from build123d import *

# Parameters (mm, degrees)
BOSS_EXTRUDE2_DEPTH = 10
SKETCH3_R           = 3.5
BOSS_EXTRUDE3_DEPTH = 60
SKETCH4_R           = 3.5
BOSS_EXTRUDE4_DEPTH = 10


with BuildPart() as part:
    # Sketch1 → Boss-Extrude2 (new body)
    with BuildSketch(Plane.XY):
        with BuildLine():
            Line((0, 22.75), (0, -22.75))
            ThreePointArc((0, -22.75), (-0.292893219, -23.457106781), (-1, -23.75))
            Line((-1, -23.75), (-29, -23.75))
            ThreePointArc((-29, -23.75), (-29.707106781, -23.457106781), (-30, -22.75))
            Line((-30, -22.75), (-30, -14.75))
            ThreePointArc((-30, -14.75), (-29.707106781, -14.042893219), (-29, -13.75))
            Line((-29, -13.75), (-11, -13.75))
            ThreePointArc((-11, -13.75), (-10.292893219, -13.457106781), (-10, -12.75))
            Line((-10, -12.75), (-10, 32.75))
            ThreePointArc((-10, 32.75), (-9.707106781, 33.457106781), (-9, 33.75))
            Line((-9, 33.75), (19, 33.75))
            ThreePointArc((19, 33.75), (19.707106781, 33.457106781), (20, 32.75))
            Line((20, 32.75), (20, 24.75))
            ThreePointArc((20, 24.75), (19.707106781, 24.042893219), (19, 23.75))
            Line((19, 23.75), (1, 23.75))
            ThreePointArc((1, 23.75), (0.292893219, 23.457106781), (0, 22.75))
        make_face()
    extrude(amount=BOSS_EXTRUDE2_DEPTH)

    # Sketch3 → Boss-Extrude3 (add)
    with BuildSketch(Plane(origin=(20, 0, 0), x_dir=(0, 0, -1), z_dir=(1, 0, 0))):
        with Locations(Location((-5, 28.75, 0), (0, 0, 270))):
            Circle(SKETCH3_R)
    extrude(amount=BOSS_EXTRUDE3_DEPTH)

    # Sketch4 → Boss-Extrude4 (add)
    with BuildSketch(Plane.ZY.offset(30)):
        with Locations(Location((5, -18.75, 0), (0, 0, 90))):
            Circle(SKETCH4_R)
    extrude(amount=BOSS_EXTRUDE4_DEPTH)


solid = part.part
Work out the finished part from the listing and answer in its coordinate system (mm). A direction names the side the tool comes from. Round coordinates to 2 decimals unless told otherwise and drop trailing zeros. Write each loop counter-clockwise with the first axis right and the second up, starting at its lowest first coordinate (ties: lowest second). Pieces come first, ordered by that corner, then holes. Notation, with made-up numbers: (75, 19.5) - (80, 19.5) arc R15 ccw to (80, 35.5) - close; hole circle Ø8 at (15, -10.75). An arc over 180 degrees is marked (long way). Answer in a Markdown table with one row per item. Add a question column.
1. A cutting plane is placed at D-D, the plane x = 40. Determine the outline of the cut face in (y, z), and give its area (3 significant figures).
2. For faces 1 (the flat face through (0, 0, 5)), 2 (the cylindrical face through (-34.9, -15.5, 6.3)), 3 (the cylindrical face through (49.58, 25.41, 3.95)), 4 (the flat face through (-20, -13.75, 5)), determine the directions among +Z, -Z, +X, -X, +Y, -Y from which every point of the face is accessible in a straight line to the end or side of a thin tool.
3. A cutting plane is placed at A-A, the plane y = -18.75. Determine the outline of the cut face in (x, z).
4. A cutting plane is placed at C-C, the plane y = 28.75. Determine the outline of the cut face in (x, z).
5. A cutting plane is placed at B-B, the plane z = 5. Determine the outline of the cut face in (x, y), and give its area (3 significant figures).
6. Find the intervals of material crossed by line 1 along Y through (x, z) = (-11, 9); line 2 along X through (y, z) = (7, 9.75); line 3 along Y through (x, z) = (2.5, 1.75), in increasing order. Write a range as from..to.
7. Given pin 1 (10 mm diameter, centred on x = 4, y = -5.5, fed in from +Z); pin 2 (1 mm diameter, centred on x = 59.5, z = 6.5, fed in from +Y); pin 3 (3 mm diameter, centred on y = 3.5, z = 5, fed in from +X); pin 4 (5 mm diameter, centred on y = 16.5, z = 3, fed in from -X), each flat-ended and moving along its own axis, determine where each tip first touches the part or whether it passes through.
Worked out:
| question | item | result |
|---|---|---|
| 1 | outline | circle Ø7 at (28.75, 5) |
| 1 | area | 38.5 mm^2 |
| 2 | face 1 | +Z, -Z, +X, -Y |
| 2 | face 2 | -X |
| 2 | face 3 | +X |
| 2 | face 4 | +Z, -Z, -X, +Y |
| 3 | outline | (-40, 1.5) - (-30, 1.5) - (-30, 0) - (0, 0) - (0, 10) - (-30, 10) - (-30, 8.5) - (-40, 8.5) - close |
| 4 | outline | (-10, 0) - (20, 0) - (20, 1.5) - (80, 1.5) - (80, 8.5) - (20, 8.5) - (20, 10) - (-10, 10) - close |
| 5 | outline | (-40, -22.25) - (-30, -22.25) - (-30, -22.75) arc R1 ccw to (-29, -23.75) - (-1, -23.75) arc R1 ccw to (0, -22.75) - (0, 22.75) arc R1 cw to (1, 23.75) - (19, 23.75) arc R1 ccw to (20, 24.75) - (20, 25.25) - (80, 25.25) - (80, 32.25) - (20, 32.25) - (20, 32.75) arc R1 ccw to (19, 33.75) - (-9, 33.75) arc R1 ccw to (-10, 32.75) - (-10, -12.75) arc R1 cw to (-11, -13.75) - (-29, -13.75) arc R1 ccw to (-30, -14.75) - (-30, -15.25) - (-40, -15.25) - close |
| 5 | area | 1,460 mm^2 |
| 6 | line 1 | -23.75..-13.75 |
| 6 | line 2 | -10..0 |
| 6 | line 3 | 23.75..33.75 |
| 7 | pin 1 | z = 10 |
| 7 | pin 2 | y = 32.1 |
| 7 | pin 3 | x = 0 |
| 7 | pin 4 | x = -10 |
